```python
from build123d import *

# Parameters (mm, degrees)
SKETCH_10_W         = 15
SKETCH_10_H         = 8
EXTRUDE_7_DEPTH     = 41
CUT_EXTRUDE_4_DEPTH = 11
SKETCH_12_W         = 15
SKETCH_12_H         = 6
EXTRUDE_8_DEPTH     = 6
SKETCH_14_W         = 15
SKETCH_14_H         = 5
EXTRUDE_9_DEPTH     = 4
EXTRUDE_10_DEPTH    = 15
EXTRUDE_11_DEPTH    = 5
SKETCH_19_R         = 1.1
CUT_EXTRUDE_5_DEPTH = 5
EXTRUDE_START       = 0.5
SKETCH_20_R         = 1.5
SKETCH_20_R_2       = 1.1
EXTRUDE_12_DEPTH    = 0.5
SKETCH_21_R         = 1.5
SKETCH_21_R_2       = 1.1
EXTRUDE_13_DEPTH    = 0.5
FILLET_4_R          = 0.5
CHAMFER_1_SIZE      = 4.493554602
CHAMFER_1_SIZE_2    = 2.7
FILLET_7_R          = 2
SKETCH_23_W         = 15
SKETCH_23_H         = 2
CUT_EXTRUDE_6_DEPTH = 30
FILLET_8_R          = 10
FILLET_9_R          = 5
FILLET_10_R         = 2


# Some blends are built 0.0001 mm under size
with BuildPart() as part:
    # 草图10 → 凸台-拉伸7 (new body)
    with BuildSketch(Plane.XY):
        with Locations((0, 24.68211788)):
            Rectangle(SKETCH_10_W, SKETCH_10_H)
    extrude(amount=EXTRUDE_7_DEPTH)

    # 草图11 → 切除-拉伸4 (cut)
    with BuildSketch(Plane(origin=(0, 28.68211788, 0), x_dir=(1, 0, 0), z_dir=(0, 1, 0))):
        with BuildLine():
            Line((-3.45, -4), (-3.45, -6))
            ThreePointArc((-3.45, -6), (-5, -7.55), (-6.55, -6))
            Line((-6.55, -6), (-6.55, -4))
            ThreePointArc((-6.55, -4), (-5, -2.45), (-3.45, -4))
        make_face()
        with BuildLine():
            Line((3.45, -4), (3.45, -6))
            ThreePointArc((3.45, -6), (5, -7.55), (6.55, -6))
            Line((6.55, -6), (6.55, -4))
            ThreePointArc((6.55, -4), (5, -2.45), (3.45, -4))
        make_face()
    extrude(amount=-CUT_EXTRUDE_4_DEPTH, mode=Mode.SUBTRACT)

    # 草图12 → 凸台-拉伸8 (add)
    with BuildSketch(Plane.XY.offset(41)):
        with Locations((0, 25.68211788)):
            Rectangle(SKETCH_12_W, SKETCH_12_H)
    extrude(amount=EXTRUDE_8_DEPTH)

    # 草图14 → 凸台-拉伸9 (add)
    with BuildSketch(Plane.XY.offset(47)):
        with Locations((0, 23.5)):
            Rectangle(SKETCH_14_W, SKETCH_14_H)
    extrude(amount=EXTRUDE_9_DEPTH)

    # 草图17 → 凸台-拉伸10 (add)
    with BuildSketch(Plane.ZY.offset(7.5)):
        Polygon((51, 26), (54.535533906, 29.535533906), (58.071067812, 26), (53.071067812, 21), (51, 21), align=None)
    extrude(amount=-EXTRUDE_10_DEPTH)

    # 草图18 → 凸台-拉伸11 (add)
    with BuildSketch(Plane(origin=(0, -16.035533906, 16.035533906), x_dir=(1, 0, 0), z_dir=(0, -0.7071067811865507, 0.7071067811865445))):
        with BuildLine():
            Line((7.5, 59.447222151), (-7.5, 59.447222151))
            ThreePointArc((-7.5, 59.447222151), (0, 66.947222151), (7.5, 59.447222151))
        make_face()
    extrude(amount=-EXTRUDE_11_DEPTH)

    # 草图19 → 切除-拉伸5 (cut)
    with BuildSketch(Plane(origin=(0, -16.035533906, 16.035533906), x_dir=(1, 0, 0), z_dir=(0, -0.7071067811865507, 0.7071067811865445))):
        with Locations(Location((0, 59.447222151, 0), (0, 0, 270))):
            Circle(SKETCH_19_R)
    extrude(amount=-CUT_EXTRUDE_5_DEPTH, mode=Mode.SUBTRACT)

    # 草图20 → 凸台-拉伸12 (add)
    with BuildSketch(Plane(origin=(0, -16.035533906, 16.035533906), x_dir=(1, 0, 0), z_dir=(0, -0.7071067811865507, 0.7071067811865445)).offset(EXTRUDE_START)):
        with Locations(Location((0, 59.447222151, 0), (0, 0, 270))):
            Circle(SKETCH_20_R)
        with Locations(Location((0, 59.447222151, 0), (0, 0, 270))):
            Circle(SKETCH_20_R_2, mode=Mode.SUBTRACT)
    extrude(amount=-EXTRUDE_12_DEPTH)

    # 草图21 → 凸台-拉伸13 (add)
    with BuildSketch(Plane(origin=(0, -12.5, 12.5), x_dir=(1, 0, 0), z_dir=(0, 0.7071067811865513, -0.7071067811865437))):
        with Locations(Location((0, -59.447222151, 0), (0, 0, 90))):
            Circle(SKETCH_21_R)
        with Locations(Location((0, -59.447222151, 0), (0, 0, 90))):
            Circle(SKETCH_21_R_2, mode=Mode.SUBTRACT)
    extrude(amount=EXTRUDE_13_DEPTH)

    # 圆角4
    fillet_4_edges = [part.edges().sort_by_distance(p)[0] for p in [
        (0, 27.060660172, 59.131727984),
        (0, 30.596194078, 55.596194078),
    ]]
    fillet(fillet_4_edges, radius=FILLET_4_R - 0.0001)  # a hair under: the kernel refuses the full size

    # 倒角1
    # the kernel refuses this chamfer: 4.493554602, 2.7 mm, written as the material it adds along each edge
    with BuildSketch(Plane(origin=(-7.5, 26, 47), x_dir=(0, -0.019914630580833353, 0.9998016840798123), z_dir=(1, 0, 0))) as chamfer_1_piece_1_section:
        Polygon((CHAMFER_1_SIZE * 0.999801684157, -CHAMFER_1_SIZE * 0.0199146305824), (-CHAMFER_1_SIZE_2 * 0.0199146305808, -CHAMFER_1_SIZE_2 * 0.99980168408), (0, 0), align=None)
    chamfer_1_piece_1 = extrude(amount=15, mode=Mode.PRIVATE)
    chamfer_1_piece_1 = split(chamfer_1_piece_1, bisect_by=Plane(origin=(0, 28.68211788, 48.477199106), z_dir=(0, -1, 0)), keep=Keep.TOP, mode=Mode.PRIVATE)
    add(chamfer_1_piece_1)

    # 圆角7
    fillet_7_edges = [part.edges().sort_by_distance(p)[0] for p in [
        (0, 26.18524881, 51.18524881),
        (0, 28.68211788, 47.029760846),
    ]]
    fillet(fillet_7_edges, radius=FILLET_7_R)

    # 草图23 → 切除-拉伸6 (cut)
    with BuildSketch(Plane.XY.offset(41)):
        with Locations((0, 21.68211788)):
            Rectangle(SKETCH_23_W, SKETCH_23_H)
    extrude(amount=-CUT_EXTRUDE_6_DEPTH, mode=Mode.SUBTRACT)

    # 圆角8
    # the kernel refuses this fillet: 10 mm, written as the material it adds along each edge
    with BuildSketch(Plane(origin=(7.5, 22.68211788, 11), x_dir=(0, -1, 0), z_dir=(-1, 0, 0))) as fillet_8_piece_1:
        with BuildLine():
            CenterArc((10, 6), FILLET_8_R, 180, 36.869897646)
            Line((0, 6), (-0.2, 6))
            Line((-0.2, 6), (-0.2, 0))
            Line((-0.2, 0), (0, -0.2))
            ThreePointArc((0, -0.2), (1, -0.2), (1.84, -0.12))
            Line((1.84, -0.12), (2, 0))
        make_face()
    extrude(amount=15)
    with BuildSketch(Plane(origin=(7.5, 22.68211788, 47), x_dir=(0, 0, -1), z_dir=(-1, 0, 0))) as fillet_8_piece_2:
        with BuildLine():
            CenterArc((5.550931186, 10), FILLET_8_R, 236.282871199, 33.717128801)
            Line((0, 1.68211788), (-0.111018624, 1.515760238))
            ThreePointArc((-0.111018624, 1.515760238), (-0.2, 0.84105894), (-0.2, 0))
            Line((-0.2, 0), (0, -0.2))
            Line((0, -0.2), (5.550931186, -0.2))
            Line((5.550931186, -0.2), (5.550931186, 0))
        make_face()
    extrude(amount=15)

    # 圆角9
    fillet_9_edges = [part.edges().sort_by_distance(p)[0] for p in [
        (0, 20.68211788, 11),
        (0, 21, 47),
        (0, 21, 53.071067812),
    ]]
    fillet(fillet_9_edges, radius=FILLET_9_R)

    # 圆角10
    fillet_10_edges = [part.edges().sort_by_distance(p)[0] for p in [
        (0, 28.68211788, 0),
    ]]
    fillet(fillet_10_edges, radius=FILLET_10_R)


solid = part.part
```
Geometry: final body of the model. Coordinates: model frame, mm. A direction names the side the tool comes from. Round coordinates to 2 decimals unless told otherwise and drop trailing zeros. Write each loop counter-clockwise with the first axis right and the second up, starting at its lowest first coordinate (ties: lowest second). Pieces come first, ordered by that corner, then holes. Notation, with made-up numbers: (72.25, -15.75) -> (77.25, -15.75) arc R28 ccw to (77.25, 6.25) -> close; hole circle Ø11 at (-35.75, -17). An arc over 180 degrees is marked (long way). Return JSON: item names as keys, results as strings.
Q1. Section C-C on z = 24. Return the cut outline in (x, y), and give its area (3 significant figures).
From the geometry:
{"outline": "(-7.5, 22.68) -> (7.5, 22.68) -> (7.5, 28.68) -> (-7.5, 28.68) -> close", "area": "90.0 mm2"}
Q2. Set-up query: faces 1 (the flat face through (0, 20.682, 5)), 2 (the flat face through (7.5, 25, 29)), 3 (the cylindrical face through (5.03, 24.74, 2.45)), 4 (the flat face through (-0.105, 27.683, 48.692)), 5 (the flat face through (0, 22.682, 29)). Return all of +Z, -Z, +X, -X, +Y, -Y with unobstructed straight access to the full face (end or side cutting, diameter ignored); none if empty.
From the geometry:
{"face 1": "+Z, -Z, +X, -X, -Y", "face 2": "+Z, -Z, +X, +Y, -Y", "face 3": "+Y, -Y", "face 4": "+X, -X, +Y", "face 5": "+X, -X, -Y"}
Q3. Ray query, line 1 (Y direction, x = -1, z = 34.5); line 2 (Z direction, x = 5.75, y = 21.75); line 3 (Z direction, x = 0, y = 21.75). Return the intervals inside material, ascending.
From the geometry:
{"line 1": "22.68 to 28.68", "line 2": "0 to 2.64, 7.36 to 12.78, 45.66 to 53.63", "line 3": "0 to 12.78, 45.66 to 53.63"}
Q4. Section B-B on y = 23.5. Return the cut outline in (x, z), and give its area (3 significant figures).
From the geometry:
{"outline": "(-7.5, 0) -> (7.5, 0) -> (7.5, 55.57) -> (-7.5, 55.57) -> close; hole (-6.55, 4) arc R1.55 ccw to (-3.45, 4) -> (-3.45, 6) arc R1.55 ccw to (-6.55, 6) -> close; hole (3.45, 4) arc R1.55 ccw to (6.55, 4) -> (6.55, 6) arc R1.55 ccw to (3.45, 6) -> close", "area": "806 mm2"}
Q5. First-contact query: pin 1 Ø5 at (x, y) = (-0.5, 28) entering from +Z; pin 2 Ø3 at (x, z) = (-2, 56) entering from -Y; pin 3 Ø2 at (x, z) = (1, 14.5) entering from +Y. Flat tips, straight axial feed; report the tip coordinate or a pass-through.
From the geometry:
{"pin 1": "z = 62.57", "pin 2": "y = 22.43", "pin 3": "y = 28.68"}
Q6. Mould query, pull axis Y, two halves, no side actions, for faces 6 (the flat face through (6.55, 25, 5)), 7 (the cylindrical face through (-0.048, 28.515, 57.11)), 8 (the cylindrical face through (0.105, 28.607, 47.017)). Classes: +Y half, -Y half, draft (parallel to the pull), parting line (faces both ways), or undercut.
From the geometry:
{"face 6": "draft", "face 7": "undercut", "face 8": "+Y half"}
Q7. Section A-A on x = 4.25. Return the cut outline in (y, z).
From the geometry:
{"outline": "(20.68, 0) -> (26.68, 0) arc R2 ccw to (28.68, 2) -> (28.68, 2.64) -> (20.68, 2.64) -> close; (20.68, 7.36) -> (28.68, 7.36) -> (28.68, 46.48) arc R2 ccw to (28.4, 47.51) -> (26.99, 49.85) arc R2 cw to (27.29, 52.29) -> (33.91, 58.91) -> (30.37, 62.44) -> (22.46, 54.54) arc R5 ccw to (21, 51) -> (21, 48.35) arc R5 ccw to (21.56, 46.05) arc R10 cw to (22.68, 41.45) -> (22.68, 17) arc R10 cw to (21.35, 12.01) arc R5 ccw to (20.68, 9.52) -> close"}
Q8. Section D-D on x = -6. Return the cut outline in (y, z), and give its area (3 significant figures).
From the geometry:
{"outline": "(20.68, 0) -> (26.68, 0) arc R2 ccw to (28.68, 2) -> (28.68, 2.82) -> (20.68, 2.82) -> close; (20.68, 7.18) -> (28.68, 7.18) -> (28.68, 46.48) arc R2 ccw to (28.4, 47.51) -> (26.99, 49.85) arc R2 cw to (27.29, 52.29) -> (32.72, 57.72) -> (29.18, 61.25) -> (22.46, 54.54) arc R5 ccw to (21, 51) -> (21, 48.35) arc R5 ccw to (21.56, 46.05) arc R10 cw to (22.68, 41.45) -> (22.68, 17) arc R10 cw to (21.35, 12.01) arc R5 ccw to (20.68, 9.52) -> close", "area": "358 mm2"}
